```python
from build123d import *

# Parameters (mm, degrees)
F1_DEPTH = 10.16
F2_R     = 12.675969
F3_DEPTH = 12.7


with BuildPart() as f1:
    # F0 (on Right) → F1 (new body)
    with BuildSketch(Plane.YZ):
        with BuildLine():
            ThreePointArc((0, -12.7), (8.980256, -8.980256), (12.7, 0))
            ThreePointArc((12.7, 0), (8.980256, 8.980256), (0, 12.7))
            ThreePointArc((0, 12.7), (-0.436122, 12.686768), (-0.872122, 12.67002))
            ThreePointArc((-0.872122, 12.67002), (-12.695008, -0.356034), (-0.160643, -12.698984))
            ThreePointArc((-0.160643, -12.698984), (-0.080321, -12.699491), (0, -12.7))
        make_face()
        with BuildLine():
            ThreePointArc((0, 12.7), (8.980256, 8.980256), (12.7, 0))
            ThreePointArc((12.7, 0), (8.980256, -8.980256), (0, -12.7))
            ThreePointArc((0, -12.7), (26.221595, -5.929824), (45.877051, 12.7))
            ThreePointArc((45.877051, 12.7), (22.938525, 12.832797), (0, 12.7))
        make_face()
        with BuildLine():
            ThreePointArc((-0.160643, -12.698984), (-12.695008, -0.356034), (-0.872122, 12.67002))
            ThreePointArc((-0.872122, 12.67002), (-25.79747, 5.372395), (-44.45, -12.7))
            ThreePointArc((-44.45, -12.7), (-22.305323, -12.629463), (-0.160643, -12.698984))
        make_face()
    extrude(amount=F1_DEPTH)

    # F2 (on face) → F3 (join)
    with BuildSketch(Plane.YZ.offset(10.16)):
        with Locations((1.427051, 0)):
            Circle(F2_R)
    extrude(amount=-F3_DEPTH)


solid = f1.part
```
Geometry: final body of the model. Coordinates: model frame, mm. A direction names the side the tool comes from. Round coordinates to 2 decimals unless told otherwise and drop trailing zeros. Write each loop counter-clockwise with the first axis right and the second up, starting at its lowest first coordinate (ties: lowest second). Pieces come first, ordered by that corner, then holes.
Item 1: Section query A-A (z = 0). Return loops of the section in (x, y), plus the area to 3 significant figures.
Item 2: Material intervals for L1, parallel to Y at x = -1.5, z = 0.5; L2, parallel to X at y = -23, z = -7; L3, parallel to Z at x = 1.75, y = -1, sorted ascending.
Item 3: Mould query, pull axis Y, two halves, no side actions, for faces 3 (the face through (-1.25, 8.24, 10.69)), 4 (the face through (-2.54, 1, 0)), 5 (the face through (5.01, -22.62, -12.63)), 6 (the face through (5.009, -25.48, 5.556)). Classes: +Y half, -Y half, draft (parallel to the pull), parting line (faces both ways), or undercut.
Item 4: Pin query (flat end, axial travel): P1, Ø2, axis at x = 0, y = -17, coming from the +Z side; P2, Ø5, axis at x = 8, z = -2, coming from the -Y side; P3, Ø3, axis at x = 6, z = -9, coming from the +Y side. Return the tip coordinate at first contact, or that it passes through.
Item 5: Set-up query: faces 1 (the face through (5.009, 23.26, 12.833)), 2 (the face through (10.16, 0, 0)). Return all of +Z, -Z, +X, -X, +Y, -Y with unobstructed straight access to the full face (end or side cutting, diameter ignored); none if empty.
Item 6: Section query D-D (z = -9.75). Return loops of the section in (x, y).
Item 7: Section query B-B (x = 4.75). Return loops of the section in (y, z) (3 decimals).
Item 8: Section query C-C (y = 25). Return loops of the section in (x, z).
Completed:
1. outline: (-2.54, -11.25) - (0, -11.25) - (0, -33.43) - (10.16, -33.43) - (10.16, 34.84) - (0, 34.84) - (0, 14.1) - (-2.54, 14.1) - close
1. area: 758 mm2
2. L1: y = -11.24 to 14.09
2. L2: x = 0 to 10.16
2. L3: z = -12.69 to 12.66
3. face 3: parting line
3. face 4: draft
3. face 5: undercut
3. face 6: -Y half
4. P1: stops at z = 9.84
4. P2: stops at y = -38.16
4. P3: stops at y = 23.16
5. face 1: +Z, +X, -X
5. face 2: +Z, -Z, +X, +Y, -Y
6. outline: (-2.54, -6.67) - (0, -6.67) - (0, -42.47) - (10.16, -42.47) - (10.16, 17.64) - (0, 17.64) - (0, 9.53) - (-2.54, 9.53) - close
7. outline: (-44.45, -12.7) arc R3501.347 cw to (-0.161, -12.699) arc R3215.797 cw to (0, -12.7) arc R54.102 ccw to (45.877, 12.7) arc R1981.195 ccw to (0, 12.7) arc R54.113 ccw to (-0.872, 12.67) arc R54.102 ccw to start
8. outline: (0, -6.59) - (10.16, -6.59) - (10.16, 12.83) - (0, 12.83) - close
